Work out the finished part from the listing and answer in its coordinate system (mm). Face numbers are marked on the shaded views. A direction names the side the tool comes from. Give positions to 0.01 mm unless a question says otherwise; leave off trailing zeros. Loops run counter-clockwise (first coordinate to the right, second up) from the corner with the lowest first, then second, coordinate; pieces in that order, holes last. Notation, with made-up numbers: (-6.75, 2.25) - (30.25, 2.25) arc R28 cw to (30.25, 38.25) - close; hole circle Ø3 at (71, 46). An arc over 180 degrees is marked (long way). One line per item, written item: value.
from build123d import *

# Parameters (mm, degrees)
SKETCH1_W           = 20
SKETCH1_H           = 23.7
BOSS_EXTRUDE1_DEPTH = 3.175
SKETCH2_W           = 7
SKETCH2_H           = 2.3
BOSS_EXTRUDE2_DEPTH = 3.175


with BuildPart() as part:
    # Sketch1 → Boss-Extrude1 (new body)
    with BuildSketch(Plane.XY):
        with Locations((10, 11.85)):
            Rectangle(SKETCH1_W, SKETCH1_H)
    extrude(amount=BOSS_EXTRUDE1_DEPTH)

    # Sketch2 → Boss-Extrude2 (add)
    with BuildSketch(Plane.XY.offset(3.175)):
        with Locations((10.002051165, 24.85)):
            Rectangle(SKETCH2_W, SKETCH2_H)
        with Locations((10, -1.15)):
            Rectangle(SKETCH2_W, SKETCH2_H)
    extrude(amount=-BOSS_EXTRUDE2_DEPTH)


solid = part.part
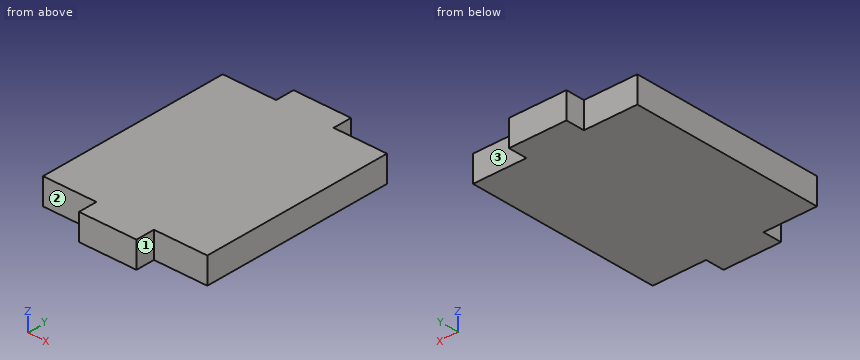
1. Find the intervals of material crossed by line 1 along X through (y, z) = (-0.5, 0.1); line 2 along Y through (x, z) = (5, 1.2), in increasing order.
Output:
line 1: x = 6.5 to 13.5
line 2: y = 0 to 23.7
2. Section A-A (z = 2.3) is taken. Write down the section's boundary in (x, y).
Output:
outline: (0, 0) - (6.5, 0) - (6.5, -2.3) - (13.5, -2.3) - (13.5, 0) - (20, 0) - (20, 23.7) - (13.5, 23.7) - (13.5, 26) - (6.5, 26) - (6.5, 23.7) - (0, 23.7) - close
3. Section B-B (x = 18.5) is taken. Write down the section's boundary in (y, z) (3 decimals).
Output:
outline: (0, 0) - (23.7, 0) - (23.7, 3.175) - (0, 3.175) - close
4. For the marked faces 1, 2 and 3, determine the directions among +Z, -Z, +X, -X, +Y, -Y from which every point of the face is accessible in a straight line to the end or side of a thin tool.
Output:
face 1: +Z, -Z, +X, -Y
face 2: +Z, -Z, -X, -Y
face 3: +Z, -Z, +X, +Y
5. Flat-ended cylindrical pins translate along their axes: pin 1 Ø1.6 at (x, z) = (15.5, 2) entering from +Y; pin 2 Ø1 at (x, z) = (15, 2.5) entering from -Y; pin 3 Ø1.8 at (y, z) = (25, 2) entering from -X. Find the tip coordinate at first contact, or state that the pin passes through.
Output:
pin 1: stops at y = 23.7
pin 2: stops at y = 0
pin 3: stops at x = 6.5
